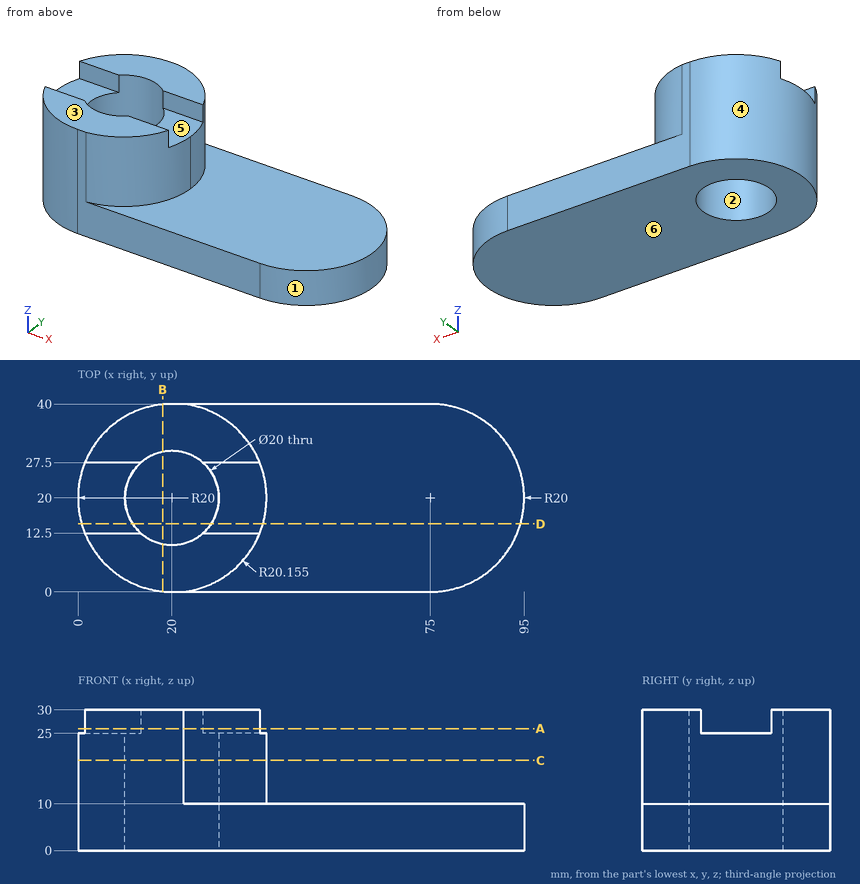
Design review of the part shown in the three views and the two pictorial views. Dimensions are in mm from the part's minimum x, y and z. A direction names the side the tool comes from. Round coordinates to 2 decimals unless told otherwise and drop trailing zeros. Write each loop counter-clockwise with the first axis right and the second up, starting at its lowest first coordinate (ties: lowest second). Pieces come first, ordered by that corner, then holes. Notation, with made-up numbers: M 38,-21 L 51,-21 A16 ccw 51,-4 Z; hole C -25.75,-38 d6. An arc over 180 degrees is marked long. One line per item, written item: value. Start each with the question number.
1. Take a section at B-B on x = 18. State the section outline as (y, z) points.
2. For the marked faces 5 and 6, list the 3-axis set-ups (+Z, -Z, +X, -X, +Y, -Y) from which the entire face can be reached by the end or side of a thin tool; tool diameter is ignored.
3. Draft analysis for pull direction X (two halves, no side actions). For the marked faces 1, 2, 3 and 4, state which applies: pulls with the +X half, pulls with the -X half, needs draft (parallel to the pull), parting line crosses it, or undercut.
4. Clearance check with flat-ended pins moving along their axes: P1, Ø12, axis at x = 72, y = 16.5, coming from the +Z side; P2, Ø5, axis at y = 35.5, z = 11.5, coming from the -X side; P3, Ø1.5, axis at x = 7, z = 28, coming from the -Y side; P4, Ø18, axis at x = 20, y = 20, coming from the -Z side. State where each tip first meets the part, or that it passes through.
5. Take a section at D-D on y = 14.5. State the section outline as (x, z) points, then the cut area to 3 significant figures.
6. Take a section at A-A on z = 26. State the section outline as (x, y) points (1 decimal).
7. To check wall thickness, follow probe 1 along X at (y, z) = (20, 22.75) (1 decimal); probe 2 along X at (y, z) = (20, 7); probe 3 along Z at (x, y) = (55, 2). State the ranges of each line that lie inside material, in increasing order. Write a range as from..to.
8. Take a section at C-C on z = 19.25. State the section outline as (x, y) points (1 decimal).
Computed:
1. outline: M 0.1,0 L 10.2,0 L 10.2,30 L 0.1,30 Z; M 29.8,0 L 39.9,0 L 39.9,30 L 29.8,30 Z
2. face 5: +Z, +X, -X
2. face 6: -Z, +X, -X, +Y, -Y
3. face 1: pulls with the +X half
3. face 2: undercut
3. face 3: needs draft
3. face 4: pulls with the -X half
4. P1: stops at z = 10
4. P2: stops at x = 4.8
4. P3: stops at y = 4.19
4. P4: passes through
5. outline: M 0.77,0 L 11.65,0 L 11.65,25 L 0.77,25 Z; M 28.35,0 L 94.23,0 L 94.23,10 L 39.39,10 L 39.39,25 L 28.35,25 Z
5. area: 1,100 mm²
6. outline: M 1.5,12.5 A20 ccw 20,0 L 22.5,0 A20.2 ccw 38.7,12.5 L 26.6,12.5 A10 cw 13.4,12.5 Z; M 1.5,27.5 L 13.4,27.5 A10 cw 26.6,27.5 L 38.7,27.5 A20.2 ccw 22.5,40 L 20,40 A20 ccw Z
7. probe 1: x = 0..10, 30..40.2
7. probe 2: x = 0..10, 30..95
7. probe 3: z = 0..10
8. outline: M 20,0 L 22.5,0 A20.2 ccw 22.5,40 L 20,40 A20 ccw Z; hole C 20,20 d20
